```python
from build123d import *

# Parameters (mm, degrees)
SKETCH3_R          = 2.3495
CUT_EXTRUDE1_DEPTH = 19.3515
FILLET1_R          = 3.175


with BuildPart() as part:
    # Sketch2 → Revolve1 (revolve)
    with BuildSketch(Plane.XY):
        Polygon((9.17575, 2.82575), (6.35, 0), (0, 0), (0, 18.3515), (6.35, 18.3515), (9.17575, 15.52575), (2.82575, 9.17575), align=None)
    revolve(axis=Axis((0, 18.3515, 0), (0, -1, 0)))

    # Sketch3 → Cut-Extrude1 (cut, through all)
    with BuildSketch(Plane(origin=(0, 18.3515, 0), x_dir=(1, 0, 0), z_dir=(0, 1, 0))):
        Circle(SKETCH3_R)
    extrude(amount=-CUT_EXTRUDE1_DEPTH, mode=Mode.SUBTRACT)

    # Fillet1
    fillet1_edges = [part.edges().sort_by_distance(p)[0] for p in [
        (-2.82575, 9.17575, 0),
    ]]
    fillet(fillet1_edges, radius=FILLET1_R)


solid = part.part
```
Input: part model. Units: mm. Frame: model coordinates. A direction names the side the tool comes from. Give positions to 0.01 mm unless a question says otherwise; leave off trailing zeros. Loops run counter-clockwise (first coordinate to the right, second up) from the corner with the lowest first, then second, coordinate; pieces in that order, holes last. Notation, with made-up numbers: M -31,21 L 28,21 A20 ccw 28,59 Z; hole C -31.75,3.25 d9. An arc over 180 degrees is marked long. Answer as CSV lines item,"result". Start each with the question number.
1. Pin query (flat end, axial travel): P1, Ø4, axis at x = 5, z = 3.5, coming from the -Y side; P2, Ø4, axis at x = 0, z = 0, coming from the +Y side; P3, Ø1, axis at x = 2, y = 11.5, coming from the -Z side; P4, Ø1, axis at x = 5, z = 7, coming from the +Y side. Return the tip coordinate at first contact, or that it passes through.
2. Line query: L1, parallel to Z at x = 0.25, y = 17; L2, parallel to Z at x = 0, y = 7; L3, parallel to X at y = 10.25, z = 0. Output: solid intervals per line, ascending.
3. Reachability of faces 1 (the face through (-1.142, 11.62, -5.145)), 2 (the face through (-1.406, 0.137, -6.333)) from +Z, -Z, +X, -X, +Y, -Y: full face, straight path, thin tool, end or side. Return the list, or none.
4. Section A-A on y = 14. Return loops of the section in (x, z), plus the area to 3 significant figures.
5. Pull-direction query (X, two-part tool) for faces 3 (the face through (-1.155, 6.674, -5.201)), 4 (the face through (3, 0, 0)), 5 (the face through (-0.31, 9.3, -2.33)); classes: released by +X, released by -X, zero draft, split by the parting line, or undercut.
6. Section B-B on y = 5.25. Return loops of the section in (x, z), plus the area to 3 significant figures.
Computed values:
1,P1,"stops at y = 0"
1,P2,"passes through"
1,P3,"stops at z = -5.31"
1,P4,"stops at y = 16.6"
2,L1,"z = -7.7 to -2.34, 2.34 to 7.7"
2,L2,"z = -5 to -2.35, 2.35 to 5"
2,L3,"x = -4.33 to -2.35, 2.35 to 4.33"
3,face 1,"none"
3,face 2,"-Y"
4,outline,"C 0,0 d15.3; hole C 0,0 d4.7"
4,area,"167 mm²"
5,face 3,"split by the parting line"
5,face 4,"zero draft"
5,face 5,"undercut"
6,outline,"C 0,0 d13.5; hole C 0,0 d4.7"
6,area,"126 mm²"
